Work out the finished part from the listing and answer in its coordinate system (mm). A direction names the side the tool comes from. Round coordinates to 2 decimals unless told otherwise and drop trailing zeros. Order: outer loops, then holes, each group sorted by start corner. A loop starts at its lowest first (then second) coordinate and runs counter-clockwise, first axis right, second up. Notation, with made-up numbers: M 1,14 L 21,14 A16 cw 21,31 Z; hole C 78,15 d2. An arc over 180 degrees is marked long. Answer as a JSON object with one key per item and string values. Group by question number.
from build123d import *

# Parameters (mm, degrees)
BOSS_EXTRUDE1_DEPTH = 30.48
SKETCH3_R           = 24.13
CUT_EXTRUDE4_DEPTH  = 90.914560616
SKETCH4_R           = 3.175
CUT_EXTRUDE5_DEPTH  = 63.754
CIRPATTERN3_COUNT   = 6
BOSS_EXTRUDE2_START = -7.62
BOSS_EXTRUDE2_DEPTH = 7.62
LPATTERN1_COUNT     = 2
LPATTERN1_PITCH     = 22.86
FILLET1_R           = 2.54


with BuildPart() as part:
    # Sketch1 → Boss-Extrude1 (new body)
    with BuildSketch(Plane(origin=(0, 0, 0), x_dir=(1, 0, 0), z_dir=(0, 1, 0))):
        with BuildLine():
            Line((-78.958715675, 0), (-17.998715675, 0))
            ThreePointArc((-17.998715675, 0), (-48.478715675, 30.349942827), (-78.958715675, 0))
        make_face()
    extrude(amount=BOSS_EXTRUDE1_DEPTH)

    # Sketch3 → Cut-Extrude4 (cut, through all)
    with BuildSketch(Plane(origin=(0, 0, 0), x_dir=(1, 0, 0), z_dir=(0, 1, 0))):
        with Locations((-48.478715675, 0)):
            Circle(SKETCH3_R)
    extrude(amount=CUT_EXTRUDE4_DEPTH, mode=Mode.SUBTRACT)

    # Sketch4 → Cut-Extrude5 (cut)
    with BuildSketch(Plane.XY):
        with Locations((-48.824364134, 15.798935299)):
            Circle(SKETCH4_R)
    cut_extrude5 = extrude(amount=-CUT_EXTRUDE5_DEPTH, mode=Mode.SUBTRACT)

    # CirPattern3: Cut-Extrude5 ×6 about axis
    cirpattern3_axis = Axis((-48.478715675, 30.48, 0.130335837), (0, -1, 0))
    for i in range(1, CIRPATTERN3_COUNT):
        add(cut_extrude5.rotate(cirpattern3_axis, i * 360 / CIRPATTERN3_COUNT), mode=Mode.SUBTRACT)

    # Sketch5 → Boss-Extrude2 (add)
    with BuildSketch(Plane(origin=(0, 30.48, 0), x_dir=(1, 0, 0), z_dir=(0, 1, 0)).offset(BOSS_EXTRUDE2_START)):
        with BuildLine():
            Line((-17.998715675, 0), (-17.236715675, 0))
            ThreePointArc((-17.236715675, 0), (-11.432288754, -3.246284223), (-11.704767509, 3.398675405))
            Line((-11.704767509, 3.398675405), (-17.236715675, 6.201452036))
            Line((-17.236715675, 6.201452036), (-18.252715675, 6.201452036))
            Line((-18.252715675, 6.201452036), (-18.663353029, 6.201452036))
            ThreePointArc((-18.663353029, 6.201452036), (-18.171997096, 3.117770752), (-17.998715675, 0))
        make_face()
        with BuildLine():
            ThreePointArc((-10.886715675, 0), (-13.426715675, -2.54), (-15.966715675, 0))
            ThreePointArc((-15.966715675, 0), (-13.426715675, 2.54), (-10.886715675, 0))
        make_face(mode=Mode.SUBTRACT)
    boss_extrude2 = extrude(amount=BOSS_EXTRUDE2_DEPTH)

    # LPattern1: Boss-Extrude2 ×2
    with Locations(*[(0, -i * LPATTERN1_PITCH, 0) for i in range(1, LPATTERN1_COUNT)]):
        add(boss_extrude2)

    # Fillet1
    fillet1_edges = [part.edges().sort_by_distance(p)[0] for p in [
        (-48.478715675, 30.48, -24.13),
    ]]
    fillet(fillet1_edges, radius=FILLET1_R)


solid = part.part
Item 1: Find section B-B (y = 18). Give the vertices of the cut face in (x, z), and give its area (3 significant figures).
Item 2: Find section C-C (x = -14). Give the vertices of the cut face in (y, z), and give its area (3 significant figures).
Item 3: Find section A-A (y = 6.5). Give the vertices of the cut face in (x, z), and give its area (3 significant figures).
Item 4: The mould has two halves that part along X. Classify faces 4 (the cylindrical face through (-25.47, 12.7, -14.35)), 5 (the cylindrical face through (-47.81, 11.64, -30.343)), 6 (the flat face through (-15.2, 22.86, -2.4)): +X half, -X half, draft (parallel to the pull), parting line (faces both ways), or undercut.
Item 5: Consider L1, parallel to X at y = 5, z = -2; L2, parallel to X at y = 3, z = -0.5; L3, parallel to Y at x = -47.5, z = -26 (3 decimals). Determine where each line is inside the solid, lowest interval first.
Item 6: A tool of negligible diameter and unlimited length cuts with its end or side. For faces 1 (the cylindrical face through (-72.51, 12.7, -12.55)), 2 (the flat face through (-21, 15, 0)), 3 (the flat face through (-18, 27, -6.201)), from which of +Z, -Z, +X, -X, +Y, -Y can it reach the whole face along a straight path? Write none if from no direction.
Item 7: Each of these flat-tipped pins is pushed along its axis until it touches: pin 1 (2 mm diameter, centred on x = -22, y = 21, fed in from +Z); pin 2 (1.6 mm diameter, centred on x = -17.5, y = 26, fed in from -Z); pin 3 (1.5 mm diameter, centred on y = 26, z = -23, fed in from -X). Where does it stop, or does it pass through?
Responses:
{
 "1": {"outline": "M -78.96,0 A30.48 ccw -76.09,-12.77 L -70.61,-9.61 A24.13 cw -72.61,0 Z; M -73.85,-16.76 A30.48 ccw -51.11,-30.24 L -51.11,-23.99 A24.13 cw -68.4,-13.61 Z; M -46.54,-30.29 A30.48 ccw -23.5,-17.33 L -28.96,-14.18 A24.13 cw -46.54,-24.05 Z; M -26.63,-10.24 L -21.16,-13.4 A30.48 ccw -18,0 L -24.35,0 A24.13 cw Z", "area": "451 mm^2"},
 "2": {"outline": "M 0,-4.56 L 7.62,-4.56 L 7.62,-2.47 L 0,-2.47 Z; M 0,2.47 L 7.62,2.47 L 7.62,3.77 L 0,3.77 Z; M 22.86,-4.56 L 30.48,-4.56 L 30.48,-2.47 L 22.86,-2.47 Z; M 22.86,2.47 L 30.48,2.47 L 30.48,3.77 L 22.86,3.77 Z", "area": "51.5 mm^2"},
 "3": {"outline": "M -78.96,0 A30.48 ccw -18.66,-6.2 L -17.24,-6.2 L -11.7,-3.4 A3.81 ccw long -17.24,0 L -24.35,0 A24.13 cw -72.61,0 Z; hole C -13.43,0 d5.08", "area": "577 mm^2"},
 "4": {"face 4": "undercut", "face 5": "parting line", "face 6": "draft"},
 "5": {"L1": "x = -78.88 to -72.53, -24.43 to -14.99, -11.86 to -10.18", "L2": "x = -78.95 to -72.6, -24.35 to -15.92, -10.94 to -9.65", "L3": "y = 0 to 12.913, 18.685 to 30.395"},
 "6": {"face 1": "none", "face 2": "+Z, -X, +Y, -Y", "face 3": "-Z, +X, +Y, -Y"},
 "7": {"pin 1": "stops at z = 0", "pin 2": "stops at z = -6.2", "pin 3": "stops at x = -69.17"}
}
